Print and shaded views of the part. All mm, measured from the part's lowest x, y and z. A direction names the side the tool comes from. Give positions to 0.01 mm unless a question says otherwise; leave off trailing zeros. Write each loop counter-clockwise with the first axis right and the second up, starting at its lowest first coordinate (ties: lowest second). Pieces come first, ordered by that corner, then holes.
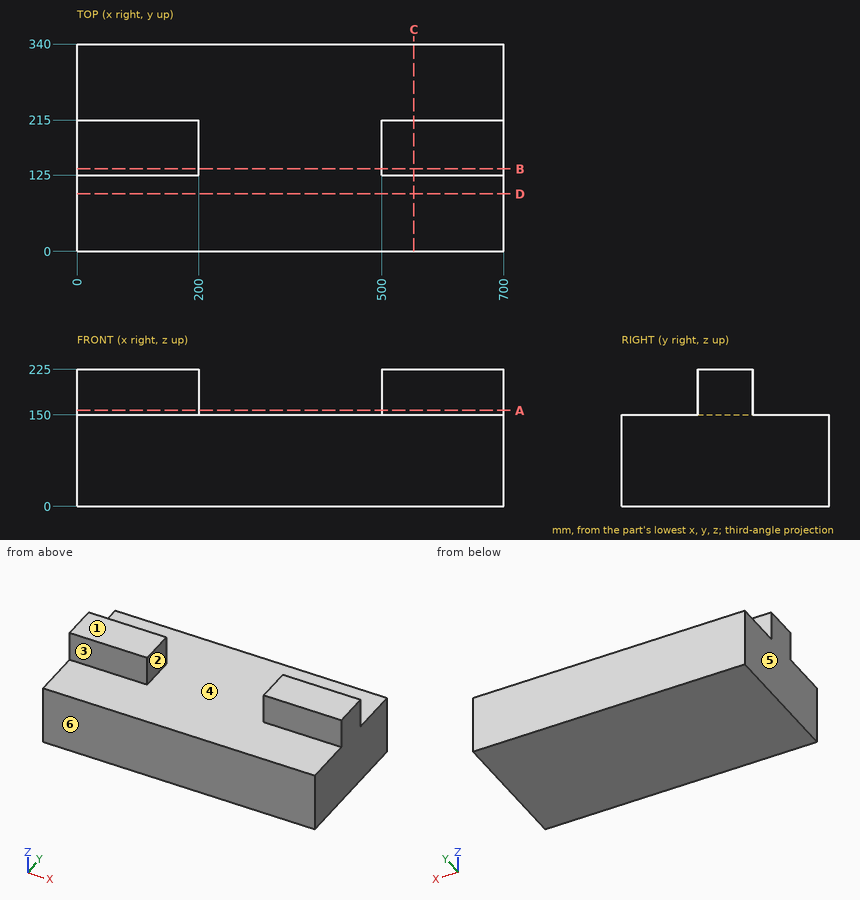
1. Saw through at A-A on z = 157.5. Give the cut face in (x, y), plus the area to 3 significant figures.
2. Saw through at D-D on y = 94. Give the cut face in (x, z).
3. 3-axis set-ups, long thin cutter, end or side, ignore diameter. For the marked faces 1, 2 and 3: which of +Z, -Z, +X, -X, +Y, -Y reach the whole face in a straight line?
4. Saw through at B-B on y = 135. Give the cut face in (x, z), plus the area to 3 significant figures.
5. Mould opens along X. For the marked faces 4, 5 and 6 say: pulls with the +X half, pulls with the -X half, needs draft (parallel to the pull), parting line crosses it, or undercut.
6. Saw through at C-C on x = 552.5. Give the cut face in (y, z), plus the area to 4 significant figures.
7. Drill centre lines: line 1 along X through (y, z) = (147.5, 207); line 2 along Y through (x, z) = (182, 165); line 3 along Z through (x, y) = (450, 117.5). Where is each one in solid material? Low to high.
8. Drop flat-ended pins along their axis: pin 1 (10 mm diameter, centred on x = 617.5, y = 268.5, fed in from -Z); pin 2 (8 mm diameter, centred on x = 461, y = 116.5, fed in from +Z); pin 3 (22.5 mm diameter, centred on x = 144.5, z = 196.5, fed in from -Y). Give the stop position or say it passes through.
Outcome:
1. outline: (0, 125) - (200, 125) - (200, 215) - (0, 215) - close; (500, 125) - (700, 125) - (700, 215) - (500, 215) - close
1. area: 36,000 mm2
2. outline: (0, 0) - (700, 0) - (700, 150) - (0, 150) - close
3. face 1: +Z, +X, -X, +Y, -Y
3. face 2: +Z, +Y, -Y
3. face 3: +Z, +X, -X, -Y
4. outline: (0, 0) - (700, 0) - (700, 225) - (500, 225) - (500, 150) - (200, 150) - (200, 225) - (0, 225) - close
4. area: 135,000 mm2
5. face 4: undercut
5. face 5: pulls with the -X half
5. face 6: needs draft
6. outline: (0, 0) - (340, 0) - (340, 150) - (215, 150) - (215, 225) - (125, 225) - (125, 150) - (0, 150) - close
6. area: 57,750 mm2
7. line 1: x = 0 to 200, 500 to 700
7. line 2: y = 125 to 215
7. line 3: z = 0 to 150
8. pin 1: stops at z = 0
8. pin 2: stops at z = 150
8. pin 3: stops at y = 125
